Here's how the part is built. I have some questions about the finished solid (model axes, mm). Face numbers are marked on the shaded views. A direction names the side the tool comes from. Round coordinates to 2 decimals unless told otherwise and drop trailing zeros. Loops run counter-clockwise (first coordinate to the right, second up) from the corner with the lowest first, then second, coordinate; pieces in that order, holes last. Notation, with made-up numbers: (-35, -30.5) -> (6, -30.5) arc R29 cw to (6, 5.5) -> close; hole circle Ø10 at (46, 15.25). An arc over 180 degrees is marked (long way). Use one line per item in the form item = value. Start each with the question number.
Item 1: If we section it at B-B (y = -97.79): Write out the boundary of the cut face in (x, z), then the cut area to 3 significant figures.
Item 2: If we section it at C-C (x = 161.29): Write out the boundary of the cut face in (y, z), then the cut area to 3 significant figures.
Item 3: If I drill on L1, parallel to Y at x = 161.29, z = 1.8; L2, parallel to X at y = -97.79, z = 0.95; L3, parallel to Y at x = 88, z = 16, over which ranges is the centre line in solid material (lowest first)? Write a range as [from, to].
Item 4: I'm going to push flat-ended pins straight in: pin 1 Ø5 at (x, z) = (97.5, 22.5) entering from -Y; pin 2 Ø1.2 at (y, z) = (-59.5, 1.5) entering from -X; pin 3 Ø11.5 at (y, z) = (-55.5, 19) entering from +X. Where does each tip first touch, or does it pass through?
Item 5: Thinking about a two-plate mould opening in Y: for the marked faces 3, 4 and 5, which applies, released by +Y, released by -Y, zero draft, split by the parting line, or undercut?
Item 6: If we section it at A-A (x = 3.81): Write out the boundary of the cut face in (y, z).
Item 7: For the marked faces 1 and 2, which set-ups out of +Z, -Z, +X, -X, +Y, -Y let a thin tool reach every point of the face, with its end or its side?
Item 8: If we section it at D-D (y = -73): Write out the boundary of the cut face in (x, z).
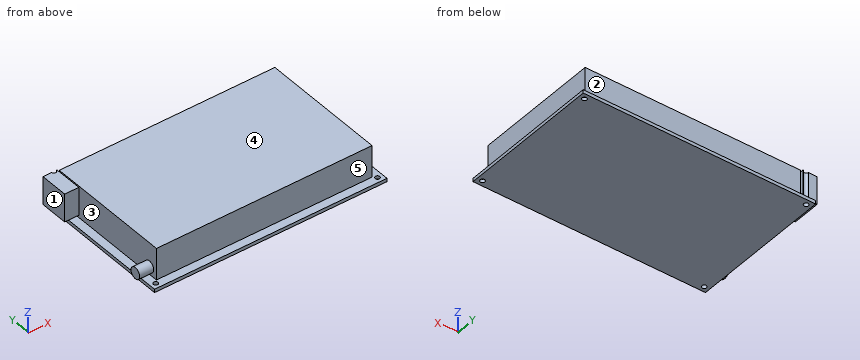
```python
from build123d import *

# Parameters (mm, degrees)
F0_W          = 153.1
F0_H          = 89.6
F1_DEPTH      = 2.4
F2_DEPTH      = 25
F3_W          = 20
F3_H          = 20
F3_R          = 4
F4_DEPTH      = 6
F4_DEPTH_BACK = 4
F5_D          = 3.3


with BuildPart() as f1:
    # F0 (on Top) → F1 (new body)
    with BuildSketch(Plane.XY):
        Polygon((165.1, 0), (0, 0), (0, -7.62), (0, -20.32), (0, -86.995), (0, -91.186), (0, -101.6), (165.1, -101.6), align=None)
        with Locations((82.55, -50.8)):
            Rectangle(F0_W, F0_H, mode=Mode.SUBTRACT)
    extrude(amount=F1_DEPTH)

    # F0 (on Top) → F2 (join)
    with BuildSketch(Plane.XY):
        with Locations((82.55, -50.8)):
            Rectangle(F0_W, F0_H)
    extrude(amount=F2_DEPTH)

    # F3 (on face) → F4 (join, two sides)
    with BuildSketch(Plane(origin=(0, 0, 0), x_dir=(0, -1, 0), z_dir=(-1, 0, 0))) as f4_sk:
        with Locations((13.97, 14)):
            Rectangle(F3_W, F3_H)
        with Locations((89.0905, 8)):
            Circle(F3_R)
    extrude(amount=-F4_DEPTH)
    extrude(f4_sk.sketch, amount=F4_DEPTH_BACK)

    # F5 (through all)
    with Locations(Plane(origin=(0, 0, 0), x_dir=(1, 0, 0), z_dir=(0, 0, -1))):
        with Locations((3.81, 3.81), (3.81, 97.79), (161.29, 97.79), (161.29, 3.81)):
            Hole(F5_D / 2)


solid = f1.part
```
Values found:
q1.outline = (0, 0) -> (2.16, 0) -> (2.16, 2.4) -> (0, 2.4) -> close; (5.46, 0) -> (159.64, 0) -> (159.64, 2.4) -> (5.46, 2.4) -> close; (162.94, 0) -> (165.1, 0) -> (165.1, 2.4) -> (162.94, 2.4) -> close
q1.area = 380 mm2
q2.outline = (-101.6, 0) -> (-99.44, 0) -> (-99.44, 2.4) -> (-101.6, 2.4) -> close; (-96.14, 0) -> (-5.46, 0) -> (-5.46, 2.4) -> (-96.14, 2.4) -> close; (-2.16, 0) -> (0, 0) -> (0, 2.4) -> (-2.16, 2.4) -> close
q2.area = 228 mm2
q3.L1 = [-101.6, -99.44], [-96.14, -5.46], [-2.16, 0]
q3.L2 = [0, 2.16], [5.46, 159.64], [162.94, 165.1]
q3.L3 = [-95.6, -6]
q4.pin_1 = -95.6
q4.pin_2 = 0
q4.pin_3 = 159.1
q5.face_3 = undercut
q5.face_4 = zero draft
q5.face_5 = released by -Y
q6.outline = (-101.6, 0) -> (-99.44, 0) -> (-99.44, 2.4) -> (-101.6, 2.4) -> close; (-96.14, 0) -> (-5.46, 0) -> (-5.46, 2.4) -> (-96.14, 2.4) -> close; circle Ø8 at (-89.09, 8); (-23.97, 4) -> (-5.46, 4) -> (-5.46, 24) -> (-23.97, 24) -> close; (-2.16, 0) -> (0, 0) -> (0, 2.4) -> (-2.16, 2.4) -> close
q7.face_1 = +Z, -Z, -X, +Y, -Y
q7.face_2 = +Z, +X, +Y
q8.outline = (0, 0) -> (165.1, 0) -> (165.1, 2.4) -> (159.1, 2.4) -> (159.1, 25) -> (6, 25) -> (6, 2.4) -> (0, 2.4) -> close
